from build123d import *

# Parameters (mm, degrees)
BOSS_EXTRUDE1_DEPTH = 50.8


with BuildPart() as part:
    # Sketch1 → Boss-Extrude1 (new body)
    with BuildSketch(Plane(origin=(0, 0, -3683), x_dir=(-1, 0, 0), z_dir=(0, 0, -1))):
        with BuildLine():
            Line((7.945265893, 3.588862728), (-1.198734107, 3.588862728))
            ThreePointArc((-1.198734107, 3.588862728), (-1.647746913, 3.774849922), (-1.833734107, 4.223862728))
            Line((-1.833734107, 4.223862728), (-1.833734107, 5.747862728))
            ThreePointArc((-1.833734107, 5.747862728), (-1.647746913, 6.196875535), (-1.198734107, 6.382862728))
            Line((-1.198734107, 6.382862728), (1.621629442, 6.382862728))
            Line((1.621629442, 6.382862728), (1.621629442, 6.890862686))
            Line((1.621629442, 6.890862686), (-2.214734107, 11.462862728))
            Line((-2.214734107, 11.462862728), (-7.294734107, 11.462862728))
            Line((-7.294734107, 11.462862728), (-11.131097656, 6.890862686))
            Line((-11.131097656, 6.890862686), (-11.131097656, 6.382862728))
            Line((-11.131097656, 6.382862728), (-8.310734107, 6.382862728))
            ThreePointArc((-8.310734107, 6.382862728), (-7.861721301, 6.196875535), (-7.675734107, 5.747862728))
            Line((-7.675734107, 5.747862728), (-7.675734107, 4.223862728))
            ThreePointArc((-7.675734107, 4.223862728), (-7.861721301, 3.774849922), (-8.310734107, 3.588862728))
            Line((-8.310734107, 3.588862728), (-17.454734107, 3.588862728))
            Line((-17.454734107, 3.588862728), (-17.727921752, 3.588862728))
            Line((-17.727921752, 3.588862728), (-17.727921752, 3.858842754))
            Line((-17.727921752, 3.858842754), (-17.728361466, 13.002372481))
            ThreePointArc((-17.728361466, 13.002372481), (-17.542256287, 13.451715967), (-17.092921752, 13.637842754))
            Line((-17.092921752, 13.637842754), (-15.568921752, 13.637842754))
            ThreePointArc((-15.568921752, 13.637842754), (-15.119908946, 13.45185556), (-14.933921752, 13.002842754))
            Line((-14.933921752, 13.002842754), (-14.933921752, 10.182479205))
            Line((-14.933921752, 10.182479205), (-14.425921794, 10.182479205))
            Line((-14.425921794, 10.182479205), (-9.853921752, 14.018842754))
            Line((-9.853921752, 14.018842754), (-9.853921752, 19.098842754))
            Line((-9.853921752, 19.098842754), (-14.425921794, 22.935206303))
            Line((-14.425921794, 22.935206303), (-14.933921752, 22.935206303))
            Line((-14.933921752, 22.935206303), (-14.933921752, 20.114842754))
            ThreePointArc((-14.933921752, 20.114842754), (-15.119908946, 19.665829948), (-15.568921752, 19.479842754))
            Line((-15.568921752, 19.479842754), (-17.092921752, 19.479842754))
            ThreePointArc((-17.092921752, 19.479842754), (-17.542476558, 19.66604812), (-17.728703542, 20.11559397))
            Line((-17.728703542, 20.11559397), (-17.728839138, 22.935206303))
            Line((-17.728839138, 22.935206303), (-21.787214199, 22.935206303))
            Line((-21.787214199, 22.935206303), (-21.791921752, 3.859128788))
            Line((-21.791921752, 3.859128788), (-21.791921752, 3.588862728))
            Line((-21.791921752, 3.588862728), (-21.791921752, -0.475137272))
            Line((-21.791921752, -0.475137272), (-17.727921752, -0.475137272))
            Line((-17.727921752, -0.475137272), (-17.454774021, -0.475137272))
            Line((-17.454774021, -0.475137272), (7.945225979, -0.475137272))
            Line((7.945225979, -0.475137272), (8.215492039, -0.475137272))
            Line((8.215492039, -0.475137272), (8.215492039, 3.588862728))
            Line((8.215492039, 3.588862728), (7.945265893, 3.588862728))
        make_face()
    extrude(amount=BOSS_EXTRUDE1_DEPTH)


solid = part.part
Check sheet for the modelled part. Datum: model origin and axes. Units: mm. A direction names the side the tool comes from. Round coordinates to 2 decimals unless told otherwise and drop trailing zeros. Loops run counter-clockwise (first coordinate to the right, second up) from the corner with the lowest first, then second, coordinate; pieces in that order, holes last.
1. Sectioned sample at B-B on y = 8.5. Record the boundary of the cut face in (x, z), and give its area (3 significant figures).
2. Gauge pin test, flat ends, axial feed: pin 1 Ø10 at (x, y) = (12.5, 6) entering from -Z; pin 2 Ø2.5 at (y, z) = (18, -3707) entering from -X; pin 3 Ø4 at (y, z) = (20, -3728) entering from +X; pin 4 Ø0.6 at (y, z) = (6.5, -3716.5) entering from -X. Record the tip position at first contact, or that the pin passes through.
3. Mould release check, pull along Y, two halves, no side actions. Record for faces 1 (the flat face through (-8.215, 2, -3708)), 2 (the flat face through (12.11, 20.99, -3708.04)), 3 (the flat face through (12.172, 12.074, -3708.044)): released by +Y, released by -Y, zero draft, split by the parting line, or undercut.
4. Sectioned sample at C-C on x = -3.5. Record the boundary of the cut face in (y, z).
5. Sectioned sample at D-D on y = 15.5. Record the boundary of the cut face in (x, z), and give its area (3 significant figures).
6. Sectioned sample at A-A on x = 10.5. Record the boundary of the cut face in (y, z), and give its area (3 significant figures).
7. Scan lines: probe 1 along X at (y, z) = (5.75, -3686); probe 2 along Y at (x, z) = (10, -3722.5); probe 3 along Y at (x, z) = (17, -3730). Record each from-to range of solid material in increasing order.
8. Set-up check for faces 4 (the flat face through (5, 11.463, -3708)), 5 (the flat face through (16, 19.48, -3708)), 6 (the flat face through (9.186, 9.209, -3708.044)): record each of +Z, -Z, +X, -X, +Y, -Y from which the full face is reachable in a straight line by a thin tool's end or side.
Recorded:
1. outline: (-0.27, -3733.8) - (9.78, -3733.8) - (9.78, -3683) - (-0.27, -3683) - close; (17.73, -3733.8) - (21.79, -3733.8) - (21.79, -3683) - (17.73, -3683) - close
1. area: 717 mm2
2. pin 1: stops at z = -3733.8
2. pin 2: stops at x = 9.85
2. pin 3: stops at x = 21.79
2. pin 4: stops at x = -1.62
3. face 1: zero draft
3. face 2: released by +Y
3. face 3: undercut
4. outline: (-0.48, -3733.8) - (3.59, -3733.8) - (3.59, -3683) - (-0.48, -3683) - close
5. outline: (9.85, -3733.8) - (21.79, -3733.8) - (21.79, -3683) - (9.85, -3683) - close
5. area: 606 mm2
6. outline: (-0.48, -3733.8) - (3.59, -3733.8) - (3.59, -3683) - (-0.48, -3683) - close; (6.38, -3733.8) - (7.64, -3733.8) - (7.64, -3683) - (6.38, -3683) - close; (13.48, -3733.8) - (19.64, -3733.8) - (19.64, -3683) - (13.48, -3683) - close
6. area: 584 mm2
7. probe 1: x = 1.83 to 7.68, 17.73 to 21.79
7. probe 2: y = -0.48 to 3.59, 6.38 to 8.24, 13.9 to 19.22
7. probe 3: y = -0.48 to 3.59, 13.64 to 19.48
8. face 4: +Z, -Z, -X, +Y
8. face 5: +Z, -Z, +Y
8. face 6: +Z, -Z
